Geometry: final body of the model. Coordinates: model frame, mm. A direction names the side the tool comes from. Coordinates: 2 decimals unless noted, no trailing zeros. Loops run counter-clockwise (first coordinate to the right, second up) from the corner with the lowest first, then second, coordinate; pieces in that order, holes last. Notation, with made-up numbers: (77.25, 87) - (136.25, 87) arc R28 ccw to (136.25, 113) - close; hole circle Ø8 at (85, -15). An arc over 180 degrees is marked (long way). Return JSON: item names as keys, results as strings.
from build123d import *
from build123d.topology import SkipClean

# Parameters (mm, degrees)
SKETCH1_W           = 4
SKETCH1_H           = 9
BOSS_EXTRUDE1_DEPTH = 25
SKETCH2_W           = 1
SKETCH2_H           = 6
CUT_EXTRUDE1_DEPTH  = 26.480384612
SKETCH4_W           = 25
SKETCH4_H           = 25
BOSS_EXTRUDE2_DEPTH = 1.5
SKETCH5_W           = 25
SKETCH5_H           = 25
BOSS_EXTRUDE3_DEPTH = 3.5
SKETCH7_W           = 1.8
SKETCH7_H           = 25
CUT_EXTRUDE5_DEPTH  = 21
CUT_EXTRUDE6_START  = -1.7
CUT_EXTRUDE6_DEPTH  = 1.7
BOSS_EXTRUDE4_START = 0.5
BOSS_EXTRUDE4_DEPTH = 0.5
SKETCH11_W          = 0.7
SKETCH11_H          = 1.5
CUT_EXTRUDE7_DEPTH  = 29.486839086
SKETCH12_W          = 1
SKETCH12_H          = 6.2
CUT_EXTRUDE8_DEPTH  = 29.486839086


with BuildPart() as part:
    # Sketch1 → Boss-Extrude1 (new body)
    with BuildSketch(Plane.XY):
        Rectangle(SKETCH1_W, SKETCH1_H)
    extrude(amount=BOSS_EXTRUDE1_DEPTH)

    # Sketch2 → Cut-Extrude1 (cut, through all)
    with BuildSketch(Plane(origin=(0, 0, 0), x_dir=(-1, 0, 0), z_dir=(0, 0, -1))):
        Rectangle(SKETCH2_W, SKETCH2_H)
    extrude(amount=-CUT_EXTRUDE1_DEPTH, mode=Mode.SUBTRACT)

    # Sketch4 → Boss-Extrude2 (add)
    with BuildSketch(Plane(origin=(2, 0, 0), x_dir=(0, 0, -1), z_dir=(1, 0, 0))):
        with Locations((-12.5, 0)):
            Rectangle(SKETCH4_W, SKETCH4_H)
    extrude(amount=-BOSS_EXTRUDE2_DEPTH)

    # Sketch5 → Boss-Extrude3 (add)
    with BuildSketch(Plane(origin=(2, 0, 0), x_dir=(0, 0, -1), z_dir=(1, 0, 0))):
        with Locations((-12.5, 0)):
            Rectangle(SKETCH5_W, SKETCH5_H)
    extrude(amount=BOSS_EXTRUDE3_DEPTH)

    # Sketch6 → Cut-Revolve2 (revolve, cut)
    with BuildSketch(Plane(origin=(0, 0, 12.5), x_dir=(-1, 0, 0), z_dir=(0, 0, -1)), mode=Mode.PRIVATE) as cut_revolve2_sk:
        with BuildLine():
            Line((-2, 10), (-2, 0))
            Line((-2, 0), (-4.699928584, 0))
            ThreePointArc((-4.699928584, 0), (-4.474492757, 5.020205958), (-3.8, 10))
            Line((-3.8, 10), (-2, 10))
        make_face()
    revolve(cut_revolve2_sk.sketch.rotate(Axis((2.075, 0, 12.5), (-1, 0, 0)), 90), axis=Axis((2.075, 0, 12.5), (-1, 0, 0)), mode=Mode.SUBTRACT)

    # Sketch7 → Cut-Extrude5 (cut)
    with BuildSketch(Plane.XZ.offset(12.5)):
        with Locations((2.9, 12.5)):
            Rectangle(SKETCH7_W, SKETCH7_H)
    extrude(amount=-CUT_EXTRUDE5_DEPTH, mode=Mode.SUBTRACT)

    # Sketch8 → Cut-Extrude6 (cut)
    with BuildSketch(Plane(origin=(5.5, 0, 0), x_dir=(0, 0, -1), z_dir=(1, 0, 0)).offset(CUT_EXTRUDE6_START)):
        with BuildLine():
            Line((-9.375, 0), (-9.375, -12.5))
            ThreePointArc((-9.375, -12.5), (-12.5, -15.625), (-15.625, -12.5))
            Line((-15.625, -12.5), (-15.625, 0))
            ThreePointArc((-15.625, 0), (-12.5, 3.125), (-9.375, 0))
        make_face()
    extrude(amount=CUT_EXTRUDE6_DEPTH, mode=Mode.SUBTRACT)

    # Sketch9 → Boss-Extrude4 (add)
    with SkipClean():  # the faces are left unmerged after this step: merging them gives an invalid solid
        with BuildSketch(Plane.ZY.offset(-3.8).offset(BOSS_EXTRUDE4_START)):
            with BuildLine():
                Line((15.625, -9.499177596), (15.625, -12.5))
                Line((15.625, -12.5), (25, -12.5))
                Line((25, -12.5), (25, 8.5))
                Line((25, 8.5), (17.767826876, 8.5))
                ThreePointArc((17.767826876, 8.5), (22.429878362, -1.182165692), (15.625, -9.499177596))
            make_face()
            with BuildLine():
                Line((0, -12.5), (9.375, -12.5))
                Line((9.375, -12.5), (9.375, -9.499177596))
                ThreePointArc((9.375, -9.499177596), (2.570121638, -1.182165692), (7.232173124, 8.5))
                Line((7.232173124, 8.5), (0, 8.5))
                Line((0, 8.5), (0, -12.5))
            make_face()
        extrude(amount=-BOSS_EXTRUDE4_DEPTH)

    # Sketch11 → Cut-Extrude7 (cut, through all)
    with SkipClean():  # the faces are left unmerged after this step: merging them gives an invalid solid
        with BuildSketch(Plane(origin=(0, 0, 0), x_dir=(-1, 0, 0), z_dir=(0, 0, -1))):
            with Locations((-0.15, -3.75)):
                Rectangle(SKETCH11_W, SKETCH11_H)
        extrude(amount=-CUT_EXTRUDE7_DEPTH, mode=Mode.SUBTRACT)

    # Sketch12 → Cut-Extrude8 (cut, through all)
    with SkipClean():  # the faces are left unmerged after this step: merging them gives an invalid solid
        with BuildSketch(Plane(origin=(0, 0, 0), x_dir=(-1, 0, 0), z_dir=(0, 0, -1))):
            Rectangle(SKETCH12_W, SKETCH12_H)
        extrude(amount=-CUT_EXTRUDE8_DEPTH, mode=Mode.SUBTRACT)


solid = part.part
Item 1: Section query B-B, the plane y = 6.25. Return loops of the section in (x, z), and give its area (3 significant figures).
Worked out:
{"outline": "(0.5, 0) - (2, 0) - (2, 25) - (0.5, 25) - close; (3.3, 0) - (5.5, 0) - (5.5, 25) - (3.3, 25) - (3.3, 20.31) - (3.8, 20.31) arc R55.66 cw to (3.8, 4.69) - (3.3, 4.69) - close", "area": "79.0 mm^2"}
Item 2: First-contact query: pin 1 Ø0.8 at (x, z) = (0, 15.5) entering from -Y; pin 2 Ø0.8 at (x, z) = (-1, 12) entering from +Y. Flat tips, straight axial feed; report the tip coordinate or a pass-through.
Worked out:
{"pin 1": "y = -4.5", "pin 2": "y = 4.5"}
Item 3: Section query D-D, the plane y = -2.75. Return loops of the section in (x, z) (3 decimals), and give its area (3 significant figures).
Worked out:
{"outline": "(-2, 0) - (-0.5, 0) - (-0.5, 25) - (-2, 25) - close; (0.5, 0) - (2, 0) - (2, 25) - (0.5, 25) - close; (3.3, 0) - (5.5, 0) - (5.5, 9.375) - (4.545, 9.375) arc R55.942 cw to (3.8, 2.886) - (3.3, 2.886) - close; (3.3, 22.114) - (3.8, 22.114) arc R55.942 cw to (4.545, 15.625) - (5.5, 15.625) - (5.5, 25) - (3.3, 25) - close", "area": "104 mm^2"}
Item 4: Mould query, pull axis Y, two halves, no side actions, for faces 6 (the face through (-1, 4.5, 12)), 7 (the face through (0, 3.1, 12)), 8 (the face through (4, -12.5, 5)), 9 (the face through (-0.2, -4, 12)). Classes: +Y half, -Y half, draft (parallel to the pull), parting line (faces both ways), or undercut.
Worked out:
{"face 6": "+Y half", "face 7": "undercut", "face 8": "-Y half", "face 9": "draft"}
Item 5: Reachability of faces 1 (the face through (5, -8, 15.625)), 2 (the face through (-0.5, 0, 12)), 3 (the face through (5.5, 3, 15)), 4 (the face through (0.5, 9, 13)), 5 (the face through (3, 8.5, 21)) from +Z, -Z, +X, -X, +Y, -Y: full face, straight path, thin tool, end or side. Return the list, or none.
Worked out:
{"face 1": "+X, -Y", "face 2": "+Z, -Z", "face 3": "+Z, -Z, +X, +Y, -Y", "face 4": "+Z, -Z, -X, +Y", "face 5": "+Z, -Z, -Y"}
Item 6: Section query C-C, the plane x = 3. Return loops of the section in (y, z), and give its area (3 significant figures).
Worked out:
{"outline": "(8.5, 0) - (12.5, 0) - (12.5, 25) - (8.5, 25) - (8.5, 17.77) arc R10 cw to (8.5, 7.23) - close", "area": "89.3 mm^2"}
Item 7: Ray query, probe 1 along Z at (x, y) = (4.5, -10.5) (3 decimals); probe 2 along X at (y, z) = (0.25, 10.75); probe 3 along X at (y, z) = (7.25, 4.5). Return the intervals inside material, ascending. Write a range as from..to.
Worked out:
{"probe 1": "0..9.375, 15.625..25", "probe 2": "-2..-0.5, 0.5..2", "probe 3": "0.5..2, 3.3..5.5"}
Item 8: Section query A-A, the plane z = 12.5. Return loops of the section in (x, y) (3 decimals).
Worked out:
{"outline": "(-2, -4.5) - (-0.2, -4.5) - (-0.2, -3.1) - (-0.5, -3.1) - (-0.5, 3.1) - (0.5, 3.1) - (0.5, -12.5) - (2, -12.5) - (2, 10) - (3.8, 10) arc R56.01 cw to (4.613, 3.125) - (5.5, 3.125) - (5.5, 12.5) - (0.5, 12.5) - (0.5, 4.5) - (-2, 4.5) - close"}
